Model file for the job. Use its own axes, mm. A direction names the side the tool comes from. Give positions to 0.01 mm unless a question says otherwise; leave off trailing zeros. Loops run counter-clockwise (first coordinate to the right, second up) from the corner with the lowest first, then second, coordinate; pieces in that order, holes last. Notation, with made-up numbers: (63.5, -6.75) - (76.5, -6.75) arc R19 ccw to (76.5, 25.25) - close; hole circle Ø3 at (-13, 76). An arc over 180 degrees is marked (long way). Answer as CSV lines item,"result". Start each with the question number.
Item 1: Saw through at A-A on z = 3. Give the cut face in (x, y).
Item 2: Drill centre lines: L1, parallel to X at y = 1.25, z = 3; L2, parallel to X at y = -0.25, z = -19.5; L3, parallel to X at y = -2.5, z = -60. Where is each one in solid material? Low to high. Write a range as from..to.
Item 3: Tool access for faces 1 (the cylindrical face through (-9.963, -0.07, 0.018)), 2 (the flat face through (0, 0, -35)): list every direction of +Z, -Z, +X, -X, +Y, -Y with a clear straight run to the whole face (end or side of a thin tool).
Item 4: Saw through at C-C on x = 1.25. Give the cut face in (y, z).
Item 5: Pull direction X, two halves, no side cores. Call faces 3 (the flat face through (0, 0, 6)), 4 (the cylindrical face through (-3.215, -0.07, 2.766)), 5 (the cylindrical face through (9.963, 0.07, 0.018)): pulls with the +X half, pulls with the -X half, needs draft (parallel to the pull), parting line crosses it, or undercut.
Item 6: Saw through at D-D on y = -1.25. State how many separate pieces and enclosed holes the cut face has, plus the area to 3 significant figures.
Item 7: Saw through at B-B on z = -10. Give the cut face in (x, y).
Item 8: Pin check, flat tips, straight feed: pin 1 (6 mm diameter, centred on x = 7, z = -51, fed in from +Y); pin 2 (6 mm diameter, centred on y = 4, z = -44, fed in from -X); pin 3 (4 mm diameter, centred on y = 4, z = -25, fed in from -X); pin 4 (0.6 mm diameter, centred on y = -0.5, z = -24.5, fed in from -X). Stop position of each tip, or through.
from build123d import *

# Parameters (mm, degrees)
SKETCH1_R           = 1.8
BOSS_EXTRUDE1_DEPTH = 5
FILLET1_R           = 15


with BuildPart() as part:
    # Sketch1 → Boss-Extrude1 (new, symmetric)
    with BuildSketch(Plane(origin=(0, 0, 0), x_dir=(1, 0, 0), z_dir=(0, 1, 0))):
        Polygon((10, -6), (10, 0), (0, 70), (-10, 0), (-10, -6), align=None)
        with Locations(Location((-5, -3, 0), (0, 0, 270))):
            Circle(SKETCH1_R, mode=Mode.SUBTRACT)
        with Locations(Location((5, -3, 0), (0, 0, 270))):
            Circle(SKETCH1_R, mode=Mode.SUBTRACT)
        Polygon((-8.918418884, 0.5), (-7.346990313, 11.5), (-5.5, 11.5), (-5.5, 11), (5.5, 11), (5.5, 11.5), (7.346990313, 11.5), (8.918418884, 0.5), (6.096000551, 0.5), (6.096000551, 1), (-5.903999449, 1), (-5.903999449, 0.5), align=None, mode=Mode.SUBTRACT)
        Polygon((-5.5, 12.5), (-7.20413317, 12.5), (-5.632704598, 23.5), (-4, 23.5), (-4, 23), (4, 23), (4, 23.5), (5.632704598, 23.5), (7.20413317, 12.5), (5.5, 12.5), (5.5, 13), (-5.5, 13), align=None, mode=Mode.SUBTRACT)
        Polygon((-4, 24.5), (-5.489847455, 24.5), (-3.918418884, 35.5), (-2.75, 35.5), (-2.75, 35), (2.75, 35), (2.75, 35.5), (3.918418884, 35.5), (5.489847455, 24.5), (4, 24.5), (4, 25), (-4, 25), align=None, mode=Mode.SUBTRACT)
        Polygon((-3.346933757, 39.500395887), (0, 62.928932188), (3.347561625, 39.496000816), (3.775561741, 36.5), (2.75, 36.5), (2.75, 37), (-2.75, 37), (-2.75, 36.5), (-3.775561741, 36.5), align=None, mode=Mode.SUBTRACT)
    extrude(amount=BOSS_EXTRUDE1_DEPTH, both=True)

    # Fillet1
    fillet1_edges = [part.edges().sort_by_distance(p)[0] for p in [
        (-10, 0, 0),
        (10, 0, 0),
    ]]
    fillet(fillet1_edges, radius=FILLET1_R)


solid = part.part
Responses:
1,outline,"(-10, -5) - (-6.8, -5) - (-6.8, 5) - (-10, 5) - close; (-3.2, -5) - (3.2, -5) - (3.2, 5) - (-3.2, 5) - close; (6.8, -5) - (10, -5) - (10, 5) - (6.8, 5) - close"
2,L1,"-10..-6.8, -3.2..3.2, 6.8..10"
2,L2,"-7.21..-6.2, 6.2..7.21"
2,L3,"-1.43..-0.42, 0.42..1.43"
3,face 1,"-Z, -X, +Y, -Y"
3,face 2,"+Y, -Y"
4,outline,"(-5, -61.25) - (5, -61.25) - (5, -54.18) - (-5, -54.18) - close; (-5, -37) - (5, -37) - (5, -35) - (-5, -35) - close; (-5, -25) - (5, -25) - (5, -23) - (-5, -23) - close; (-5, -13) - (5, -13) - (5, -11) - (-5, -11) - close; (-5, -1) - (5, -1) - (5, 6) - (-5, 6) - close"
5,face 3,"needs draft"
5,face 4,"undercut"
5,face 5,"pulls with the +X half"
6,separate pieces,"1"
6,enclosed holes,"6"
6,area,"307 mm2"
7,outline,"(-8.57, -5) - (-7.56, -5) - (-7.56, 5) - (-8.57, 5) - close; (7.56, -5) - (8.57, -5) - (8.57, 5) - (7.56, 5) - close"
8,pin 1,"through"
8,pin 2,"x = -4.14"
8,pin 3,"x = -6.71"
8,pin 4,"x = -6.54"
